```python
from build123d import *


with BuildPart() as part:
    # 草图1 → 旋转1 (revolve)
    with BuildSketch(Plane.XY, mode=Mode.PRIVATE) as revolve_1_sk:
        with BuildLine():
            Line((0, 288.881257919), (0, 0))
            Line((0, 0), (20, 0))
            Line((20, 0), (20, 100))
            Line((20, 100), (15, 100))
            Line((15, 100), (15, 200))
            Line((15, 200), (465, 200))
            Line((465, 200), (465, 240))
            Line((465, 240), (15, 240))
            Line((15, 240), (15, 290))
            ThreePointArc((15, 290), (7.520830803, 289.161331306), (0, 288.881257919))
        make_face()
        with BuildLine():
            Line((0, 390), (0, 290))
            Line((0, 290), (15, 290))
            ThreePointArc((15, 290), (76.6217369, 324.014324021), (101.118742081, 390))
            ThreePointArc((101.118742081, 390), (71.50174823, 461.50174823), (0, 491.118742081))
            Line((0, 491.118742081), (0, 390))
        make_face()
        with BuildLine():
            Line((0, 290), (0, 288.881257919))
            ThreePointArc((0, 288.881257919), (7.520830803, 289.161331306), (15, 290))
            Line((15, 290), (0, 290))
        make_face()
    revolve(revolve_1_sk.sketch.rotate(Axis((0, 290, 0), (0, 1, 0)), 90), axis=Axis((0, 290, 0), (0, 1, 0)))


solid = part.part
```
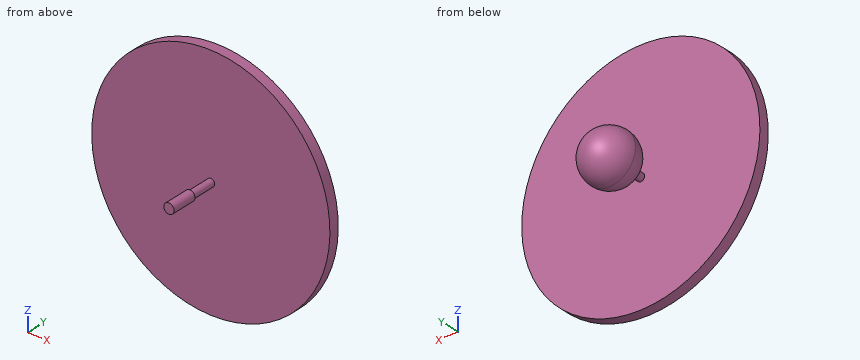
Design review of the part built by this model. Coordinates are the model's own, in mm. Coordinates: 2 decimals unless noted, no trailing zeros. Order: outer loops, then holes, each group sorted by start corner. A loop starts at its lowest first (then second) coordinate and runs counter-clockwise, first axis right, second up.
1) Clearance check with flat-ended pins moving along their axes: pin 1 (5 mm diameter, centred on x = -4, z = -57.5, fed in from +Y); pin 2 (4 mm diameter, centred on x = 103, z = 265, fed in from +Y); pin 3 (10 mm diameter, centred on x = 15.5, z = -117, fed in from -Y). State where each tip first meets the part, or that it passes through.
2) Wall thickness on line 1 along Y through (x, z) = (368.5, 211); line 2 along Y through (x, z) = (57, -37); line 3 along Z through (x, y) = (-70.5, 414.5): over which ranges is each line inside the solid? List them lowest first.
3) Take a section at D-D, the plane y = 83.5. Give the boundary of the cut face in (x, z).
4) Take a section at A-A, the plane x = 0. Give the boundary of the cut face in (y, z).
5) Take a section at C-C, the plane y = 166.5. Give the boundary of the cut face in (x, z).
6) Take a section at B-B, the plane z = 0. Give the boundary of the cut face in (x, y), and give its area (3 significant figures).
Returned:
1. pin 1: stops at y = 474.76
1. pin 2: stops at y = 240
1. pin 3: stops at y = 200
2. line 1: y = 200 to 240
2. line 2: y = 200 to 240, 315.12 to 464.88
2. line 3: z = -68.22 to 68.22
3. outline: circle Ø40 at (0, 0)
4. outline: (0, -20) - (100, -20) - (100, -15) - (200, -15) - (200, -465) - (240, -465) - (240, -15) - (290, -15) arc R101.12 ccw (long way) to (290, 15) - (240, 15) - (240, 465) - (200, 465) - (200, 15) - (100, 15) - (100, 20) - (0, 20) - close
5. outline: circle Ø30 at (0, 0)
6. outline: (-465, 200) - (-15, 200) - (-15, 100) - (-20, 100) - (-20, 0) - (20, 0) - (20, 100) - (15, 100) - (15, 200) - (465, 200) - (465, 240) - (15, 240) - (15, 290) arc R101.12 ccw (long way) to (-15, 290) - (-15, 240) - (-465, 240) - close
6. area: 77,800 mm2
